Here's how the part is built. I have some questions about the finished solid (model axes, mm). Face numbers are marked on the shaded views. A direction names the side the tool comes from. Give positions to 0.01 mm unless a question says otherwise; leave off trailing zeros. Loops run counter-clockwise (first coordinate to the right, second up) from the corner with the lowest first, then second, coordinate; pieces in that order, holes last. Notation, with made-up numbers: (51.25, 76) - (61.25, 76) arc R21 cw to (61.25, 85) - close; hole circle Ø1 at (79, 6). An arc over 180 degrees is marked (long way). Use a Markdown table: item, result.
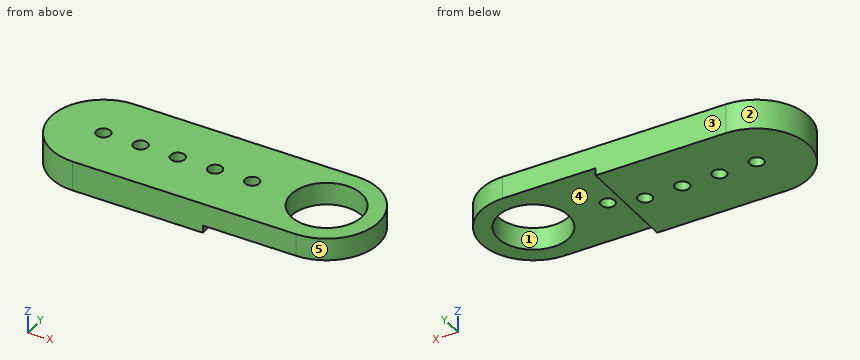
from build123d import *

# Parameters (mm, degrees)
ESQUISSE1_R             = 9.5
ESQUISSE1_R_2           = 1.9
BOSS_EXTRU_1_DEPTH      = 8
ESQUISSE3_W             = 39
ESQUISSE3_H             = 28
ENL_V_MAT_EXTRU_1_DEPTH = 2


with BuildPart() as part:
    # Esquisse1 → Boss.-Extru.1 (new body)
    with BuildSketch(Plane.XY):
        with BuildLine():
            Line((0, 14), (-60, 14))
            ThreePointArc((-60, 14), (-74, 0), (-60, -14))
            Line((-60, -14), (0, -14))
            ThreePointArc((0, -14), (14, 0), (0, 14))
        make_face()
        Circle(ESQUISSE1_R, mode=Mode.SUBTRACT)
        with Locations((-60, 0)):
            Circle(ESQUISSE1_R_2, mode=Mode.SUBTRACT)
        with Locations((-50, 0)):
            Circle(ESQUISSE1_R_2, mode=Mode.SUBTRACT)
        with Locations((-40, 0)):
            Circle(ESQUISSE1_R_2, mode=Mode.SUBTRACT)
        with Locations((-30, 0)):
            Circle(ESQUISSE1_R_2, mode=Mode.SUBTRACT)
        with Locations((-20, 0)):
            Circle(ESQUISSE1_R_2, mode=Mode.SUBTRACT)
    extrude(amount=BOSS_EXTRU_1_DEPTH)

    # Esquisse3 → Enlèv. mat.-Extru.1 (cut)
    with BuildSketch(Plane(origin=(0, 0, 0), x_dir=(-1, 0, 0), z_dir=(0, 0, -1))):
        with Locations((5.5, 0)):
            Rectangle(ESQUISSE3_W, ESQUISSE3_H)
    extrude(amount=-ENL_V_MAT_EXTRU_1_DEPTH, mode=Mode.SUBTRACT)


solid = part.part
(1) Will these pins go through, and if not, where does the flat tip stop? pin 1 (1 mm diameter, centred on y = 1.5, z = 1, fed in from +X); pin 2 (4 mm diameter, centred on y = 4.5, z = 4.5, fed in from +X) (3 decimals); pin 3 (4.5 mm diameter, centred on x = -60, y = 0, fed in from +Z); pin 4 (5 mm diameter, centred on x = -20, y = 0, fed in from -Z).
A:
| item | result |
|---|---|
| pin 1 | x = -25 |
| pin 2 | x = 13.775 |
| pin 3 | z = 8 |
| pin 4 | z = 2 |
(2) On a 3-axis mill with a long thin cutter (end or side, diameter ignored), from which of +Z, -Z, +X, -X, +Y, -Y can I reach the whole of each face in a straight line? I mean the marked faces 4 and 5. Say none if no direction works.
A:
| item | result |
|---|---|
| face 4 | -Z, +X, +Y, -Y |
| face 5 | +Z, -Z, +X |
(3) Suppose I cut it at C-C on z = 3.25. Write out the boundary of the cut face in (x, y).
A:
| item | result |
|---|---|
| outline | (-60, -14) - (0, -14) arc R14 ccw to (0, 14) - (-60, 14) arc R14 ccw to start; hole circle Ø3.8 at (-60, 0); hole circle Ø3.8 at (-50, 0); hole circle Ø3.8 at (-40, 0); hole circle Ø3.8 at (-30, 0); hole circle Ø3.8 at (-20, 0); hole circle Ø19 at (0, 0) |
(4) Suppose I cut it at D-D on x = -2.5. Write out the boundary of the cut face in (y, z).
A:
| item | result |
|---|---|
| outline | (-14, 2) - (-9.17, 2) - (-9.17, 8) - (-14, 8) - close; (9.17, 2) - (14, 2) - (14, 8) - (9.17, 8) - close |
(5) If I drill on line 1 (Y direction, x = -40, z = 4); line 2 (Y direction, x = 0, z = 4.65); line 3 (X direction, y = -1, z = 1), over which ranges is the centre line in solid material (lowest first)?
A:
| item | result |
|---|---|
| line 1 | -14 to -1.9, 1.9 to 14 |
| line 2 | -14 to -9.5, 9.5 to 14 |
| line 3 | -73.96 to -61.62, -58.38 to -51.62, -48.38 to -41.62, -38.38 to -31.62, -28.38 to -25 |
(6) Suppose I cut it at B-B on y = 7.5. Write out the boundary of the cut face in (x, z), plus the area to 3 significant figures.
A:
| item | result |
|---|---|
| outline | (-71.82, 0) - (-25, 0) - (-25, 2) - (-5.83, 2) - (-5.83, 8) - (-71.82, 8) - close; (5.83, 2) - (11.82, 2) - (11.82, 8) - (5.83, 8) - close |
| area | 526 mm2 |
(7) Suppose I cut it at A-A on x = -50. Write out the boundary of the cut face in (y, z).
A:
| item | result |
|---|---|
| outline | (-14, 0) - (-1.9, 0) - (-1.9, 8) - (-14, 8) - close; (1.9, 0) - (14, 0) - (14, 8) - (1.9, 8) - close |
(8) We'd pull the mould along X, two halves only. Please class the marked faces 1, 2 and 3: pulls with the +X half, pulls with the -X half, needs draft (parallel to the pull), parting line crosses it, or undercut.
A:
| item | result |
|---|---|
| face 1 | undercut |
| face 2 | pulls with the -X half |
| face 3 | needs draft |
